The model under review builds one solid part; all positions refer to its coordinate system, in mm. Give positions to 0.01 mm unless a question says otherwise; leave off trailing zeros. Loops run counter-clockwise (first coordinate to the right, second up) from the corner with the lowest first, then second, coordinate; pieces in that order, holes last. Notation, with made-up numbers: (7.5, 68) - (49.5, 68) arc R21 cw to (49.5, 86) - close; hole circle Ø9 at (-20, -23.5). An arc over 180 degrees is marked (long way). Return JSON: item names as keys, results as strings. Group by question number.
```python
from build123d import *

# Parameters (mm, degrees)
SKETCH1_W           = 187.7087417
SKETCH1_H           = 180
SKETCH1_W_2         = 14
SKETCH1_H_2         = 10
SKETCH1_W_3         = 12.5
SKETCH1_W_4         = 5
SKETCH1_H_3         = 15
SKETCH1_W_5         = 10
SKETCH1_H_4         = 5
SKETCH1_R           = 7.5
SKETCH1_W_6         = 15
BOSS_EXTRUDE1_DEPTH = 10


with BuildPart() as part:
    # Sketch1 → Boss-Extrude1 (new body)
    with BuildSketch(Plane.XY):
        Rectangle(SKETCH1_W, SKETCH1_H)
        with Locations((-71.95437085, -68.7)):
            Rectangle(SKETCH1_W_2, SKETCH1_H_2, mode=Mode.SUBTRACT)
        with Locations((-42.95437085, -68.7)):
            Rectangle(SKETCH1_W_2, SKETCH1_H_2, mode=Mode.SUBTRACT)
        with Locations((-43.75, -32.5)):
            Rectangle(SKETCH1_W_3, SKETCH1_H_2, mode=Mode.SUBTRACT)
        with Locations((-18.35, -13.8)):
            Rectangle(SKETCH1_W_4, SKETCH1_H_3, mode=Mode.SUBTRACT)
        with Locations((0, -85.5)):
            Rectangle(SKETCH1_W_5, SKETCH1_H_4, mode=Mode.SUBTRACT)
        with Locations((0, -68.7)):
            Circle(SKETCH1_R, mode=Mode.SUBTRACT)
        with Locations((42.95437085, -68.7)):
            Rectangle(SKETCH1_W_2, SKETCH1_H_2, mode=Mode.SUBTRACT)
        with Locations((71.95437085, -68.7)):
            Rectangle(SKETCH1_W_2, SKETCH1_H_2, mode=Mode.SUBTRACT)
        with Locations((0, -32.5)):
            Rectangle(SKETCH1_W_3, SKETCH1_H_2, mode=Mode.SUBTRACT)
        with Locations((43.75, -32.5)):
            Rectangle(SKETCH1_W_3, SKETCH1_H_2, mode=Mode.SUBTRACT)
        Circle(SKETCH1_R, mode=Mode.SUBTRACT)
        with Locations((-18.35, 9.2)):
            Rectangle(SKETCH1_W_4, SKETCH1_H_3, mode=Mode.SUBTRACT)
        with Locations((-43.75, 32.5)):
            Rectangle(SKETCH1_W_3, SKETCH1_H_2, mode=Mode.SUBTRACT)
        with Locations((-18.35, 32.2)):
            Rectangle(SKETCH1_W_4, SKETCH1_H_3, mode=Mode.SUBTRACT)
        with Locations((-71.95437085, 68.7)):
            Rectangle(SKETCH1_W_2, SKETCH1_H_2, mode=Mode.SUBTRACT)
        with Locations((-42.95437085, 68.7)):
            Rectangle(SKETCH1_W_2, SKETCH1_H_2, mode=Mode.SUBTRACT)
        with Locations((0, 32.5)):
            Rectangle(SKETCH1_W_3, SKETCH1_H_2, mode=Mode.SUBTRACT)
        with Locations((43.75, 32.5)):
            Rectangle(SKETCH1_W_3, SKETCH1_H_2, mode=Mode.SUBTRACT)
        with Locations((2.65, 54.7)):
            Rectangle(SKETCH1_W_6, SKETCH1_H_2, mode=Mode.SUBTRACT)
        with Locations((25.65, 54.7)):
            Rectangle(SKETCH1_W_6, SKETCH1_H_2, mode=Mode.SUBTRACT)
        with Locations((0, 85.5)):
            Rectangle(SKETCH1_W_5, SKETCH1_H_4, mode=Mode.SUBTRACT)
        with Locations((42.95437085, 68.7)):
            Rectangle(SKETCH1_W_2, SKETCH1_H_2, mode=Mode.SUBTRACT)
        with Locations((48.65, 54.7)):
            Rectangle(SKETCH1_W_6, SKETCH1_H_2, mode=Mode.SUBTRACT)
        with Locations((71.95437085, 68.7)):
            Rectangle(SKETCH1_W_2, SKETCH1_H_2, mode=Mode.SUBTRACT)
    extrude(amount=BOSS_EXTRUDE1_DEPTH)


solid = part.part
```
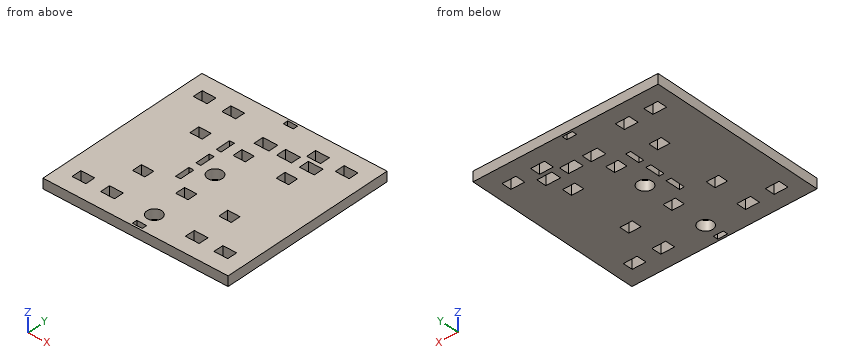
1) We need section C-C, the plane x = 22. Write out the cut boundary in (y, z), plus the area to 3 significant figures.
2) We need section D-D, the plane y = -68.7. Write out the cut boundary in (x, z).
3) To check wall thickness, follow line 1 (X direction, y = -32, z = 7.75); line 2 (Y direction, x = -38, z = 2.5); line 3 (Y direction, x = 37, z = 2). State the ranges of each line that lie inside material, in increasing order.
4) We need section A-A, the plane y = 54. Write out the cut boundary in (x, z), plus the area to 3 significant figures.
5) We need section B-B, the plane x = 0. Count the separate pieces of the cut face and the enclosed holes in it, plus the area to 3 significant figures.
Findings:
{
 "1": {"outline": "(-90, 0) - (49.7, 0) - (49.7, 10) - (-90, 10) - close; (59.7, 0) - (90, 0) - (90, 10) - (59.7, 10) - close", "area": "1,700 mm^2"},
 "2": {"outline": "(-93.85, 0) - (-78.95, 0) - (-78.95, 10) - (-93.85, 10) - close; (-64.95, 0) - (-49.95, 0) - (-49.95, 10) - (-64.95, 10) - close; (-35.95, 0) - (-7.5, 0) - (-7.5, 10) - (-35.95, 10) - close; (7.5, 0) - (35.95, 0) - (35.95, 10) - (7.5, 10) - close; (49.95, 0) - (64.95, 0) - (64.95, 10) - (49.95, 10) - close; (78.95, 0) - (93.85, 0) - (93.85, 10) - (78.95, 10) - close"},
 "3": {"line 1": "x = -93.85 to -50, -37.5 to -6.25, 6.25 to 37.5, 50 to 93.85", "line 2": "y = -90 to -73.7, -63.7 to -37.5, -27.5 to 27.5, 37.5 to 63.7, 73.7 to 90", "line 3": "y = -90 to -73.7, -63.7 to 63.7, 73.7 to 90"},
 "4": {"outline": "(-93.85, 0) - (-4.85, 0) - (-4.85, 10) - (-93.85, 10) - close; (10.15, 0) - (18.15, 0) - (18.15, 10) - (10.15, 10) - close; (33.15, 0) - (41.15, 0) - (41.15, 10) - (33.15, 10) - close; (56.15, 0) - (93.85, 0) - (93.85, 10) - (56.15, 10) - close", "area": "1,430 mm^2"},
 "5": {"separate pieces": "8", "enclosed holes": "0", "area": "1,100 mm^2"}
}
